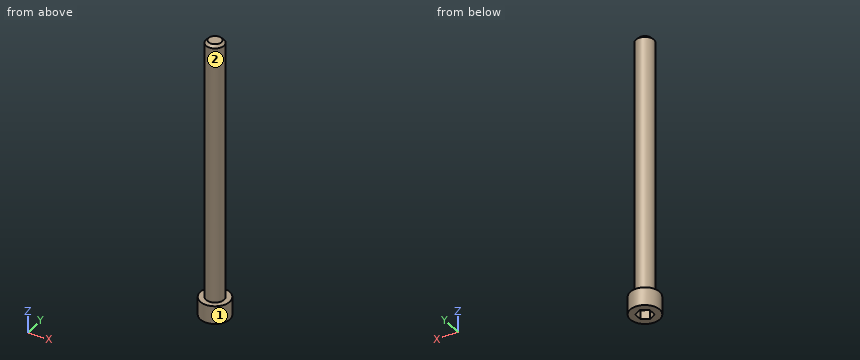
Autodesk Inventor part; units mm, degrees
ref_plane "YZ Plane" through (0, 0, 0) normal (1, 0, 0) x (0, 1, 0)
ref_plane "XZ Plane" through (0, 0, 0) normal (0, 1, 0) x (-1, 0, 0)
ref_plane "XY Plane" through (0, 0, 0) normal (0, 0, 1) x (1, 0, 0)
sketch "Sketch1" plane through (0, 0, 0) normal (0, 0, 1) x (1, 0, 0)
  circle A0 centre (0, 0) radius 1.7526
  dimension "d0" = 3.5052
extrude "Extrusion1" add sketch "Sketch1" along normal blind 50.8
sketch "Sketch2" plane through (0, 0, 0) normal (0, 0, -1) x (-1, 0, 0)
  circle A0 centre (0, 0) radius 1.7526 construction
  circle A1 centre (0, 0) radius 2.8702
  dimension "d3" = 5.7404
extrude "Extrusion2" add sketch "Sketch2" along normal blind 3.5052
sketch "Sketch3" plane through (0, 0, -3.5052) normal (0, 0, -1) x (-1, 0, 0)
  circle A0 centre (0, 0) radius 2.8702
  line L0 (0, 1.604) -> (1.3891, 0.802)
  line L1 (1.3891, 0.802) -> (1.3891, -0.802)
  line L2 (1.3891, -0.802) -> (0, -1.604)
  line L3 (0, -1.604) -> (-1.3891, -0.802)
  line L4 (-1.3891, -0.802) -> (-1.3891, 0.802)
  line L5 (-1.3891, 0.802) -> (0, 1.604)
  dimension "d6" = 2.7781
extrude "Extrusion3" cut sketch "Sketch3" against normal blind 1.7526 contours L0 L1 L2 L3 L4 L5
chamfer "Chamfer1" distance 0.508 angle 45 1 edges at (-1.7526, 0, 50.8)
thread "Thread2"
properties part number "6-32 SHCS x500" material "Stainless Steel"
Input: part model. Units: mm. Frame: model coordinates. Face numbers are marked on the shaded views. A direction names the side the tool comes from. Coordinates: 2 decimals unless noted, no trailing zeros. Order: outer loops, then holes, each group sorted by start corner. A loop starts at its lowest first (then second) coordinate and runs counter-clockwise, first axis right, second up.
1. Contact query for flat-ended pins moving along their axis: P1, Ø1.5, axis at x = 1, y = 1.5, coming from the +Z side; P2, Ø2, axis at y = 0, z = 22.5, coming from the -X side. Output: stop coordinate, or through.
Checked values:
P1: stops at z = 50.8
P2: stops at x = -1.75
2. Ray query, line 1 along Y through (x, z) = (0, 9); line 2 along Z through (x, y) = (-1.55, 0.9). Return the intervals inside material, ascending.
Checked values:
line 1: y = -1.75 to 1.75
line 2: z = -3.51 to 0
3. Cut plane B-B, the plane z = 35. Return loops of the section in (x, y).
Checked values:
outline: circle Ø3.51 at (0, 0)
4. Cut plane A-A, the plane y = 0. Return loops of the section in (x, z).
Checked values:
outline: (-2.87, -3.51) - (-1.39, -3.51) - (-1.39, -1.75) - (1.39, -1.75) - (1.39, -3.51) - (2.87, -3.51) - (2.87, 0) - (1.75, 0) - (1.75, 50.29) - (1.24, 50.8) - (-1.24, 50.8) - (-1.75, 50.29) - (-1.75, 0) - (-2.87, 0) - close
5. Access query for the marked faces 1 and 2. Directions: +Z, -Z, +X, -X, +Y, -Y. A direction counts if a zero-diameter tool reaches every point of the face in a straight line with its end or side. Return the directions, or none.
Checked values:
face 1: +Z, -Z
face 2: +Z
